Geometry: final body of the model. Coordinates: model frame, mm. A direction names the side the tool comes from. Give positions to 0.01 mm unless a question says otherwise; leave off trailing zeros. Order: outer loops, then holes, each group sorted by start corner. A loop starts at its lowest first (then second) coordinate and runs counter-clockwise, first axis right, second up. Notation, with made-up numbers: (-11, -27) - (39, -27) arc R13 ccw to (39, -21) - close; hole circle Ø8 at (42, -29). An arc over 180 degrees is marked (long way). One line per item, written item: value.
```python
from build123d import *

# Parameters (mm, degrees)
F0_R          = 20
F1_DEPTH      = 100
F2_W          = 60
F2_H          = 60
F3_DEPTH      = 30
F3_DEPTH_BACK = 40
F4_W          = 15
F4_H          = 20
F5_DEPTH      = 380
F6_W          = 15
F6_H          = 50
F7_DEPTH      = 50
F8_R          = 20
F9_DEPTH      = 75.001
F11_DEPTH     = 75.001
F13_DEPTH     = 100.001
F14_R         = 25
F15_DEPTH     = 8
F16_W         = 60
F16_H         = 35
F17_DEPTH     = 2
F18_W         = 60
F18_H         = 42
F19_DEPTH     = 2
F20_W         = 60
F20_H         = 35
F21_DEPTH     = 2
F22_W         = 60
F22_H         = 40
F23_DEPTH     = 2


with BuildPart() as f1:
    # F0 (on Right) → F1 (new body)
    with BuildSketch(Plane.YZ):
        Circle(F0_R)
    extrude(amount=F1_DEPTH)

    # F2 (on Front) → F3 (join, two sides)
    with BuildSketch(Plane.XZ) as f3_sk:
        with Locations((45, 0)):
            Rectangle(F2_W, F2_H)
    extrude(amount=F3_DEPTH)
    extrude(f3_sk.sketch, amount=-F3_DEPTH_BACK)

    # F4 (on face) → F5 (join)
    with BuildSketch(Plane.XZ.offset(30)):
        with Locations((67.5, 20)):
            Rectangle(F4_W, F4_H)
        with Locations((22.5, 20)):
            Rectangle(F4_W, F4_H)
        with Locations((22.5, -20)):
            Rectangle(F4_W, F4_H)
        with Locations((67.5, -20)):
            Rectangle(F4_W, F4_H)
    extrude(amount=F5_DEPTH)

    # F6 (on face) → F7 (join)
    with BuildSketch(Plane.XY.offset(30)):
        with Locations((67.5, -385)):
            Rectangle(F6_W, F6_H)
        with Locations((22.5, -385)):
            Rectangle(F6_W, F6_H)
    extrude(amount=-F7_DEPTH)

    # F8 (on face) → F9 (cut, through all)
    with BuildSketch(Plane.YZ.offset(75)):
        with Locations((-385, 0)):
            Circle(F8_R)
    extrude(amount=-F9_DEPTH, mode=Mode.SUBTRACT)

    # F10 (on face) → F11 (cut, through all)
    with BuildSketch(Plane.YZ.offset(75)):
        with BuildLine():
            ThreePointArc((-380, -30), (-410, 0), (-380, 30))
            Line((-380, 30), (-431.153561, 30))
            Line((-431.153561, 30), (-431.153561, -30))
            Line((-431.153561, -30), (-380, -30))
        make_face()
    extrude(amount=-F11_DEPTH, mode=Mode.SUBTRACT)

    # F12 (on Right) → F13 (cut, through all)
    with BuildSketch(Plane.YZ):
        with BuildLine():
            ThreePointArc((0, 30), (29.527362, 0.003723), (0, -29.992553))
            Line((0, -29.992553), (38.263392, -57.712726))
            Line((38.263392, -57.712726), (73.062226, -4.995079))
            Line((73.062226, -4.995079), (49.949568, 52.137349))
            Line((49.949568, 52.137349), (0, 30))
        make_face()
    extrude(amount=F13_DEPTH, mode=Mode.SUBTRACT)

    # F14 (on face) → F15 (join)
    with BuildSketch(Plane.YZ.offset(75)):
        Circle(F14_R)
    extrude(amount=F15_DEPTH)

    # F16 (on face) → F17 (join)
    with BuildSketch(Plane.XY.offset(-10)):
        with Locations((45, -47.5)):
            Rectangle(F16_W, F16_H)
    extrude(amount=-F17_DEPTH)

    # F18 (on face) → F19 (join)
    with BuildSketch(Plane.XZ.offset(65)):
        with Locations((45, 9)):
            Rectangle(F18_W, F18_H)
    extrude(amount=-F19_DEPTH)

    # F20 (on face) → F21 (join)
    with BuildSketch(Plane.XY.offset(-10)):
        with Locations((45, -342.5)):
            Rectangle(F20_W, F20_H)
    extrude(amount=-F21_DEPTH)

    # F22 (on face) → F23 (join)
    with BuildSketch(Plane(origin=(0, -325, 0), x_dir=(-1, 0, 0), z_dir=(0, 1, 0))):
        with Locations((-45, 10)):
            Rectangle(F22_W, F22_H)
    extrude(amount=-F23_DEPTH)


solid = f1.part
```
1) Mould query, pull axis Z, two halves, no side actions, for faces 1 (the face through (30, -217, -14)), 2 (the face through (22, -193, -10)), 3 (the face through (91.381, -4.336, -19.524)). Classes: released by +Z, released by -Z, zero draft, split by the parting line, or undercut.
Answers below:
face 1: zero draft
face 2: undercut
face 3: split by the parting line
2) Material intervals for line 1 along Y through (x, z) = (42.5, -1); line 2 along X through (y, z) = (-50, 17); line 3 along Z through (x, y) = (72, -307), sorted ascending.
Answers below:
line 1: -327 to -325, -65 to -63, -30 to 29.51
line 2: 15 to 30, 60 to 75
line 3: -30 to -10, 10 to 30
3) Section A-A, the plane y = -344. Return loops of the section in (x, z), then the cut area to 3 significant figures.
Answers below:
outline: (15, -30) - (30, -30) - (30, -12) - (60, -12) - (60, -30) - (75, -30) - (75, -10) - (15, -10) - close; (15, 10) - (30, 10) - (30, 30) - (15, 30) - close; (60, 10) - (75, 10) - (75, 30) - (60, 30) - close
area: 1,260 mm^2
4) Section D-D, the plane z = 0. Count the separate pieces of the cut face and the enclosed holes in it, then the cut area to 3 significant figures.
Answers below:
separate pieces: 7
enclosed holes: 0
area: 5,790 mm^2
5) Set-up query: faces 4 (the face through (7.395, -4.336, -19.524)), 5 (the face through (22, -343, 10)), 6 (the face through (45, -63, 6)), 7 (the face through (60, -47, 20)), 8 (the face through (60, -197, 20)). Return all of +Z, -Z, +X, -X, +Y, -Y with unobstructed straight access to the full face (end or side cutting, diameter ignored); none if empty.
Answers below:
face 4: -X
face 5: +X, -X
face 6: none
face 7: +Z
face 8: +Z, -Z
6) First-contact query: pin 1 (4 mm diameter, centred on x = 41, z = 22.5, fed in from +Y); pin 2 (5 mm diameter, centred on x = 88.5, z = -12, fed in from +Y); pin 3 (4.5 mm diameter, centred on x = 24.5, z = -2.5, fed in from +Y). Flat tips, straight axial feed; report the tip coordinate or a pass-through.
Answers below:
pin 1: y = 21.43
pin 2: y = 17.6
pin 3: y = 29.53
7) Section C-C, the plane y = -117. Return loops of the section in (x, z).
Answers below:
outline: (15, -30) - (30, -30) - (30, -10) - (15, -10) - close; (15, 10) - (30, 10) - (30, 30) - (15, 30) - close; (60, -30) - (75, -30) - (75, -10) - (60, -10) - close; (60, 10) - (75, 10) - (75, 30) - (60, 30) - close
